Work out the finished part from the listing and answer in its coordinate system (mm). Coordinates: 2 decimals unless noted, no trailing zeros. Order: outer loops, then holes, each group sorted by start corner. A loop starts at its lowest first (then second) coordinate and runs counter-clockwise, first axis right, second up.
Autodesk Inventor part; units mm, degrees
ref_plane "YZ Plane" through (0, 0, 0) normal (1, 0, 0) x (0, 1, 0)
ref_plane "XZ Plane" through (0, 0, 0) normal (0, 1, 0) x (-1, 0, 0)
ref_plane "XY Plane" through (0, 0, 0) normal (0, 0, 1) x (1, 0, 0)
sketch "Sketch1" plane through (0, 0, 0) normal (0, 1, 0) x (-1, 0, 0)
  line L0 (0, 0) -> (0, -228.6)
  line L1 (0, -228.6) -> (123.5964, -228.6)
  line L2 (123.5964, -228.6) -> (123.5964, 0)
  line L3 (123.5964, 0) -> (0, 0)
  dimension "d0" = 228.6
  dimension "d1" = 123.5964
extrude "Plate1" add sketch "Sketch1" along normal blind 0.5
sketch "Sketch2" plane through (0, 0.8078, -228.206) normal (0, -0.6156615, -0.7880108) x (1, 0, 0)
  line L0 (-123.5964, 0) -> (0, 0)
  line L1 (0, 0) -> (0, 184.15)
  line L2 (0, 184.15) -> (-123.5964, 184.15)
  line L3 (-123.5964, 184.15) -> (-123.5964, 0)
edge flange "Flange1" height 184.15 angle 128 thickness 0.5 bend radius 0.5 thickness toward (0, -0.6156615, -0.7880108) relief tear relief width 0.5 relief depth 0.25 edges at (-61.7982, 0, -228.6) wall of the first edge with corners at (-123.5964, 0.8078, -228.206) (0, 0.8078, -228.206) (0, -144.3043, -114.8319) (-123.5964, -144.3043, -114.8319)
bend "Bend1"
corner "Corner1"
ref_plane "Work Plane2" through (-123.5964, 0, -114.3) normal (0, 0, -1) x (1, 0, 0)
ref_plane "Work Plane1" through (-123.5964, 0, 0) normal (0, 0, -1) x (1, 0, 0)
sketch "Sketch4" plane through (0, -144.6122, -115.2259) normal (0, -0.6156615, -0.7880108) x (-1, 0, 0)
  line L0 (0, 63.5) -> (50.8, 63.5)
  line L1 (50.8, 63.5) -> (50.8, 136.271)
  line L2 (50.8, 136.271) -> (0, 136.271)
  line L3 (0, 0) -> (0, 182.0997)
  line L4 (0, 63.5) -> (0, 136.271)
  line L5 (123.5964, 0) -> (0, 0)
  dimension "d22" = 50.8
  dimension "d23" = 63.5
  dimension "d24" = 72.771
extrude "Cut2" cut sketch "Sketch4" against normal blind 0.5
equation "\"d25\" = Thickness"
equation "\"d3\" = BendReliefWidth"
equation "\"d4\" = BendReliefDepth"
equation "\"d5\" = MinimumRemnant"
equation "\"d6\" = BendRadius"
equation "\"d9\" = BendRadius"
equation "\"d10\" = CornerReliefSize"
equation "\"d11\" = GapSize"
equation "\"d12\" = JacobiRadiusSize"
equation "\"BendRadius\" = Thickness"
equation "\"BendReliefWidth\" = Thickness"
equation "\"BendReliefDepth\" = 0.5 * Thickness"
equation "\"CornerReliefSize\" = 4 * Thickness"
equation "\"MinimumRemnant\" = 2 * Thickness"
equation "\"TransitionRadius\" = BendRadius"
equation "\"JacobiRadiusSize\" = BendRadius"
equation "\"GapSize\" = Thickness"
equation "\"d2\" = BendRadius"
properties part number "Autofeeder frame1"
1. The part is cut by section B-B (x = -111). Determine the outline of the cut face in (y, z), plus the area to 3 significant figures.
2. Consider probe 1 along Y at (x, z) = (-72, -140.5); probe 2 along Y at (x, z) = (-68.5, -79); probe 3 along Y at (x, z) = (-28, -128.5). Determine where each line is inside the solid, lowest interval first.
3. Flat-ended cylindrical pins translate along their axes: pin 1 (4 mm diameter, centred on x = -63, z = -147.5, fed in from -Y); pin 2 (12 mm diameter, centred on x = -53.5, y = -77, fed in from -Z); pin 3 (13.5 mm diameter, centred on y = -75.5, z = -168, fed in from +X). Find the tip coordinate at first contact, or state that the pin passes through.
4. The part is cut by section D-D (z = -191). Determine the outline of the cut face in (x, y).
5. The part is cut by section C-C (z = -139.5). Determine the outline of the cut face in (x, y).
6. The mould has two halves that part along Y. Classify faces 1 (the flat face through (-50.8, -66.2, -176.2)), 2 (the flat face through (-74.666, -73.868, -170.497)), 3 (the flat face through (-61, 0.5, -112)), 4 (the flat face through (-74.666, -71.552, -171.673)): released by +Y, released by -Y, zero draft, split by the parting line, or undercut.
7. The part is cut by section A-A (x = -11). Determine the outline of the cut face in (y, z), plus the area to 3 significant figures.
Worked out:
1. outline: (-144.61, -115.23) - (-1.12, -227.34) arc R1 ccw to (0.5, -226.55) - (0.5, 0) - (0, 0) - (0, -226.55) arc R0.5 cw to (-0.81, -226.94) - (-144.3, -114.83) - close
1. area: 205 mm2
2. probe 1: y = -112.26 to -111.45, 0 to 0.5
2. probe 2: y = 0 to 0.5
2. probe 3: y = -127.62 to -126.81, 0 to 0.5
3. pin 1: stops at y = -105.86
3. pin 2: stops at z = -172.74
3. pin 3: stops at x = -50.8
4. outline: (-123.6, -47.63) - (-50.8, -47.63) - (-50.8, -46.81) - (-123.6, -46.81) - close; (-123.6, 0) - (0, 0) - (0, 0.5) - (-123.6, 0.5) - close
5. outline: (-123.6, -113.54) - (0, -113.54) - (0, -112.73) - (-123.6, -112.73) - close; (-123.6, 0) - (0, 0) - (0, 0.5) - (-123.6, 0.5) - close
6. face 1: zero draft
6. face 2: released by -Y
6. face 3: released by +Y
6. face 4: undercut
7. outline: (-144.61, -115.23) - (-94.57, -154.32) - (-94.27, -153.93) - (-144.3, -114.83) - close; (-37.23, -199.12) - (-1.12, -227.34) arc R1 ccw to (0.5, -226.55) - (0.5, 0) - (0, 0) - (0, -226.55) arc R0.5 cw to (-0.81, -226.94) - (-36.92, -198.73) - close
7. area: 169 mm2
